from build123d import *

# Parameters (mm, degrees)
EXTRUDE_1_DEPTH = 20


with BuildPart() as part:
    # 草图1 → 凸台-拉伸1 (new body)
    with BuildSketch(Plane.XY):
        with BuildLine():
            Line((-102.522059495, 8.076343046), (-111.898526204, 11.122941761))
            ThreePointArc((-111.898526204, 11.122941761), (-120.809688049, 9.743554451), (-124.987713204, 1.752583259))
            ThreePointArc((-124.987713204, 1.752583259), (-125, 0), (-124.987713204, -1.752583259))
            ThreePointArc((-124.987713204, -1.752583259), (-120.809688049, -9.743554451), (-111.898526204, -11.122941761))
            Line((-111.898526204, -11.122941761), (-102.522059495, -8.076343046))
            ThreePointArc((-102.522059495, -8.076343046), (-101.136647244, -7.671824451), (-99.729424961, -7.3513126))
            ThreePointArc((-99.729424961, -7.3513126), (-100, 0), (-99.729424961, 7.3513126))
            ThreePointArc((-99.729424961, 7.3513126), (-101.136647244, 7.671824451), (-102.522059495, 8.076343046))
        make_face()
        with BuildLine():
            ThreePointArc((-106.426584774, -0.463525492), (-104.536474508, -1.426584774), (-103.573415226, 0.463525492))
            ThreePointArc((-103.573415226, 0.463525492), (-105.463525492, 1.426584774), (-106.426584774, -0.463525492))
        make_face(mode=Mode.SUBTRACT)
        with BuildLine():
            ThreePointArc((-116.426584774, -0.463525492), (-114.536474508, -1.426584774), (-113.573415226, 0.463525492))
            ThreePointArc((-113.573415226, 0.463525492), (-115.463525492, 1.426584774), (-116.426584774, -0.463525492))
        make_face(mode=Mode.SUBTRACT)
    extrude(amount=EXTRUDE_1_DEPTH)


solid = part.part
Can you work these out from the model? Positions are in its coordinate system, mm. Round coordinates to 2 decimals unless told otherwise and drop trailing zeros. Write each loop counter-clockwise with the first axis right and the second up, starting at its lowest first coordinate (ties: lowest second). Pieces come first, ordered by that corner, then holes. Notation, with made-up numbers: (51, -0.75) - (60, -0.75) arc R23 ccw to (60, 21.25) - close; hole circle Ø9 at (86.5, -16). An arc over 180 degrees is marked (long way). Write each question's results on one line, items separated by ' | '. Start each with the question number.
1) Suppose I cut it at D-D (x = -105). List the corners of the cut face in (y, z) for me.
2) We'd pull the mould along Y, two halves only. Please class faces 1 (the cylindrical face through (-100, 0, 10)), 2 (the flat face through (-113, 0, 20)), 3 (the flat face through (-107.145, 9.578, 9.86)): released by +Y, released by -Y, zero draft, split by the parting line, or undercut.
3) For pin 1 Ø1.5 at (y, z) = (6, 7) entering from +X; pin 2 Ø12 at (x, z) = (-119, 4.5) entering from +Y; pin 3 Ø1.5 at (x, z) = (-109, 15) entering from +Y; pin 4 Ø2 at (x, z) = (-105.5, 9) entering from -Y, each with a flat end and sliding along its axis, tell me the tip position at first contact or that it passes through.
4) Suppose I cut it at B-B (x = -115). List the corners of the cut face in (y, z) for me.
5) Suppose I cut it at C-C (z = 14.25). List the corners of the cut face in (x, y) for me.
6) Suppose I cut it at A-A (y = 0). List the corners of the cut face in (x, z) for me.
7) Please list where these lines run through material, in increasing order: line 1 (X direction, y = 0, z = 3); line 2 (Y direction, x = -116, z = 6.75); line 3 (X direction, y = 6.75, z = 4).
Here are the results:
1) outline: (-8.88, 0) - (-1.5, 0) - (-1.5, 20) - (-8.88, 20) - close; (1.5, 0) - (8.88, 0) - (8.88, 20) - (1.5, 20) - close
2) face 1: undercut | face 2: zero draft | face 3: released by +Y
3) pin 1: stops at x = -99.77 | pin 2: stops at y = 11.61 | pin 3: stops at y = 10.42 | pin 4: stops at y = -9.37
4) outline: (-11.61, 0) - (-1.5, 0) - (-1.5, 20) - (-11.61, 20) - close; (1.5, 0) - (11.61, 0) - (11.61, 20) - (1.5, 20) - close
5) outline: (-124.99, -1.75) arc R10 ccw to (-111.9, -11.12) - (-102.52, -8.08) arc R24 cw to (-99.73, -7.35) arc R100 cw to (-99.73, 7.35) arc R24 cw to (-102.52, 8.08) - (-111.9, 11.12) arc R10 ccw to (-124.99, 1.75) arc R125 ccw to start; hole circle Ø3 at (-115, 0); hole circle Ø3 at (-105, 0)
6) outline: (-125, 0) - (-116.5, 0) - (-116.5, 20) - (-125, 20) - close; (-113.5, 0) - (-106.5, 0) - (-106.5, 20) - (-113.5, 20) - close; (-103.5, 0) - (-100, 0) - (-100, 20) - (-103.5, 20) - close
7) line 1: x = -125 to -116.5, -113.5 to -106.5, -103.5 to -100 | line 2: y = -11.56 to -1.12, 1.12 to 11.56 | line 3: x = -123.57 to -99.77
